Design review of the part built by this model. Coordinates are the model's own, in mm. A direction names the side the tool comes from. Coordinates: 2 decimals unless noted, no trailing zeros. Order: outer loops, then holes, each group sorted by start corner. A loop starts at its lowest first (then second) coordinate and runs counter-clockwise, first axis right, second up. Notation, with made-up numbers: M 0,-29.5 L 50,-29.5 A34 cw 50,5.5 Z; hole C 80.25,-7.75 d7. An arc over 180 degrees is marked long. Use CSV: the item, a comma, the result in double quotes.
```python
from build123d import *

# Parameters (mm, degrees)
SKETCH1_W           = 22
SKETCH1_H           = 23
EXTRUDE1_DEPTH      = 6.25
EXTRUDE2_DEPTH      = 4
SKETCH3_R           = 2
EXTRUDE3_DEPTH      = 3.5
EXTRUDE4_DEPTH      = 26.11473671
FILLET1_R           = 1
SKETCH5_R           = 1
EXTRUDE5_DEPTH      = 1
SKETCH6_R           = 2.75
EXTRUDE6_DEPTH      = 0.5
EXTRUDE7_DEPTH      = 1
EXTRUDE8_DEPTH      = 33.273247435
EXTRUDE8_DEPTH_BACK = 1
EXTRUDE8_START      = -2
SKETCH8_W           = 1.5
SKETCH8_H           = 4.5
EXTRUDE9_DEPTH      = 5.75
FILLET3_R           = 0.3
FILLET4_R           = 0.5
FILLET5_R           = 2
SKETCH9_R           = 1
EXTRUDE10_DEPTH     = 11.5


with BuildPart() as part:
    # Sketch1 → Extrude1 (new, symmetric)
    with BuildSketch(Plane.XY):
        Rectangle(SKETCH1_W, SKETCH1_H)
    extrude(amount=EXTRUDE1_DEPTH, both=True)

    # Sketch2 → Extrude2 (add)
    with BuildSketch(Plane(origin=(11, 0, 0), x_dir=(0, 0, -1), z_dir=(1, 0, 0))):
        with BuildLine():
            Line((-3.25, -0.25), (-3.25, 1.00658351))
            ThreePointArc((-3.25, 1.00658351), (0, 11.5), (3.25, 1.00658351))
            Line((3.25, 1.00658351), (3.25, -0.25))
            ThreePointArc((3.25, -0.25), (0, -3.5), (-3.25, -0.25))
        make_face()
    extrude(amount=EXTRUDE2_DEPTH)

    # Sketch3 → Extrude3 (add)
    with BuildSketch(Plane(origin=(15, 0, 0), x_dir=(0, 0, -1), z_dir=(1, 0, 0))):
        with Locations(Location((0, 5.75, 0), (0, 0, 90))):
            Circle(SKETCH3_R)
    extrude(amount=EXTRUDE3_DEPTH)

    # Sketch4 → Extrude4 (cut, through all)
    with BuildSketch(Plane.XY.offset(6.25)):
        Polygon((-9, 11.5), (-11, 11.5), (-11, 7.5), align=None)
    extrude(amount=-EXTRUDE4_DEPTH, mode=Mode.SUBTRACT)

    # Fillet1
    fillet1_edges = [part.edges().sort_by_distance(p)[0] for p in [
        (13, 1.00658351, -3.25),
        (13, 1.00658351, 3.25),
        (-11, 7.5, 0),
    ]]
    fillet(fillet1_edges, radius=FILLET1_R)

    # Sketch5 → Extrude5 (add)
    with BuildSketch(Plane(origin=(15, 0, 0), x_dir=(0, 0, -1), z_dir=(1, 0, 0))):
        with Locations(Location((0, -0.25, 0), (0, 0, 90))):
            Circle(SKETCH5_R)
    extrude(amount=EXTRUDE5_DEPTH)

    # Sketch6 → Extrude6 (add)
    with BuildSketch(Plane(origin=(15, 0, 0), x_dir=(0, 0, -1), z_dir=(1, 0, 0))):
        with Locations(Location((0, 5.75, 0), (0, 0, 90))):
            Circle(SKETCH6_R)
    extrude(amount=EXTRUDE6_DEPTH)

    # Sketch7 → Extrude7 (cut)
    with BuildSketch(Plane.ZY.offset(11)):
        with BuildLine():
            Line((-5.25, -9.5), (-6.25, -9.5))
            Line((-6.25, -9.5), (-6.25, -11.5))
            Line((-6.25, -11.5), (-4.25, -11.5))
            Line((-4.25, -11.5), (-4.25, -10.5))
            ThreePointArc((-4.25, -10.5), (-4.542893219, -9.792893219), (-5.25, -9.5))
        make_face()
        with BuildLine():
            Line((6.25, -11.5), (4.25, -11.5))
            Line((4.25, -11.5), (4.25, -10.5))
            ThreePointArc((4.25, -10.5), (4.542893219, -9.792893219), (5.25, -9.5))
            Line((5.25, -9.5), (6.25, -9.5))
            Line((6.25, -9.5), (6.25, -11.5))
        make_face()
        with BuildLine():
            Line((5.25, 9.5), (6.25, 9.5))
            Line((6.25, 9.5), (6.25, 11.5))
            Line((6.25, 11.5), (4.25, 11.5))
            Line((4.25, 11.5), (4.25, 10.5))
            ThreePointArc((4.25, 10.5), (4.542893219, 9.792893219), (5.25, 9.5))
        make_face()
        with BuildLine():
            Line((-6.25, 11.5), (-4.25, 11.5))
            Line((-4.25, 11.5), (-4.25, 10.5))
            ThreePointArc((-4.25, 10.5), (-4.542893219, 9.792893219), (-5.25, 9.5))
            Line((-5.25, 9.5), (-6.25, 9.5))
            Line((-6.25, 9.5), (-6.25, 11.5))
        make_face()
    extrude(amount=-EXTRUDE7_DEPTH, mode=Mode.SUBTRACT)

    # Sketch → Extrude8 (cut, two sides: drawn at the far end of the back side and taken through both)
    with BuildSketch(Plane.ZY.offset(11).offset(EXTRUDE8_START - EXTRUDE8_DEPTH_BACK)):
        with BuildLine():
            ThreePointArc((-4.25, 10.5), (-4.542893219, 9.792893219), (-5.25, 9.5))
            Line((-5.25, 9.5), (-6.25, 9.5))
            Line((-6.25, 9.5), (-6.25, 11.5))
            Line((-6.25, 11.5), (-4.25, 11.5))
            Line((-4.25, 11.5), (-4.25, 10.5))
        make_face()
        with BuildLine():
            Line((4.25, 10.5), (4.25, 11.5))
            Line((4.25, 11.5), (6.25, 11.5))
            Line((6.25, 11.5), (6.25, 9.5))
            Line((6.25, 9.5), (5.25, 9.5))
            ThreePointArc((5.25, 9.5), (4.542893219, 9.792893219), (4.25, 10.5))
        make_face()
    extrude(amount=EXTRUDE8_DEPTH + EXTRUDE8_DEPTH_BACK, mode=Mode.SUBTRACT)

    # Sketch8 → Extrude9 (add, symmetric)
    with BuildSketch(Plane.XY):
        with Locations((6.25, 13.75)):
            Rectangle(SKETCH8_W, SKETCH8_H)
        with Locations((6.25, -13.75)):
            Rectangle(SKETCH8_W, SKETCH8_H)
    extrude(amount=EXTRUDE9_DEPTH, both=True)

    # Fillet3
    fillet3_edges = [part.edges().sort_by_distance(p)[0] for p in [
        (15, -3.5, 0),
        (15, 0.12797788, -3.25),
        (15, 11.5, 0),
        (15, 0.12797788, 3.25),
        (15, 0.936287242, -3.347329066),
        (15, 0.936287242, 3.347329066),
    ]]
    fillet(fillet3_edges, radius=FILLET3_R)

    # Fillet4
    fillet4_edges = [part.edges().sort_by_distance(p)[0] for p in [
        (1.5, 11.5, -6.25),
        (1.5, 11.5, 6.25),
        (0.5, -11.5, -6.25),
        (0.5, -11.5, 6.25),
    ]]
    fillet(fillet4_edges, radius=FILLET4_R - 0.0001)  # a hair under: the kernel refuses the full size

    # Fillet5
    fillet5_edges = [part.edges().sort_by_distance(p)[0] for p in [
        (6.25, 16, -5.75),
        (6.25, 16, 5.75),
        (6.25, -16, -5.75),
        (6.25, -16, 5.75),
    ]]
    fillet(fillet5_edges, radius=FILLET5_R)

    # Sketch9 → Extrude10 (cut)
    with BuildSketch(Plane(origin=(7, 0, 0), x_dir=(0, 0, -1), z_dir=(1, 0, 0))):
        with Locations((0, 14)):
            Circle(SKETCH9_R)
    extrude10 = extrude(amount=-EXTRUDE10_DEPTH, mode=Mode.SUBTRACT)

    # Mirror1: Extrude10 across plane
    add(extrude10.mirror(Plane.ZX), mode=Mode.SUBTRACT)


solid = part.part
```
(1) Add section A-A on x = 1. State the section outline as (y, z) points.
The answers:
outline,"M -11.5,-5.75 A0.5 ccw -11,-6.25 L 11,-6.25 A0.5 ccw 11.5,-5.75 L 11.5,5.75 A0.5 ccw 11,6.25 L -11,6.25 A0.5 ccw -11.5,5.75 Z"
(2) For faces 1 (the face through (-10, -10, -5)), 2 (the face through (-8.986, 9.801, -4.535)), 3 (the face through (12.8, -3.5, -0.1)), 4 (the face through (16.979, 4.163, -1.217)), list the 3-axis set-ups (+Z, -Z, +X, -X, +Y, -Y) from which the entire face can be reached by the end or side of a thin tool; tool diameter is ignored.
The answers:
face 1,"-Z, -X, -Y"
face 2,"-Z, -X, +Y"
face 3,"+X, -Y"
face 4,"+X"
(3) Clearance check with flat-ended pins moving along their axes: P1, Ø1, axis at x = 6.5, z = -4.5, coming from the -Y side; P2, Ø4, axis at x = -0.5, y = 12, coming from the -Z side; P3, Ø3.5, axis at x = 0.5, z = 0, coming from the -Y side; P4, Ø1, axis at y = -0.5, z = -0.5, coming from the +X side. State where each tip first meets the part, or that it passes through.
The answers:
P1,"stops at y = -15.98"
P2,"stops at z = -6.25"
P3,"stops at y = -11.5"
P4,"stops at x = 16"
(4) Wall thickness on probe 1 along Y at (x, z) = (6.4, 0); probe 2 along X at (y, z) = (13, 2.5); probe 3 along Z at (x, y) = (6.4, -14): over which ranges is each line inside the solid? List them lowest first.
The answers:
probe 1,"y = -16 to -15, -13 to 13, 15 to 16"
probe 2,"x = 5.5 to 7"
probe 3,"z = -5.75 to -1, 1 to 5.75"
(5) Add section B-B on y = 12.5. State the section outline as (x, z) points.
The answers:
outline,"M 5.5,-5.75 L 7,-5.75 L 7,5.75 L 5.5,5.75 Z"
(6) The part is to be moulded in two halves that separate along Y. For faces 5 (the face through (16, 0, 0)), 6 (the face through (6.26, 15.4, -5.18)), 7 (the face through (15.5, 7, -2)), say which applies: pulls with the +Y half, pulls with the -Y half, needs draft (parallel to the pull), parting line crosses it, or undercut.
The answers:
face 5,"needs draft"
face 6,"pulls with the +Y half"
face 7,"undercut"
